```python
from build123d import *

# Parameters (mm, degrees)
BOSS_EXTRUDE1_DEPTH  = 3
SKETCH3_R            = 2.5
CUT_EXTRUDE1_DEPTH   = 4
LPATTERN1_COUNT      = 2
LPATTERN1_PITCH      = 40
LPATTERN1_COUNT_DIR2 = 2
LPATTERN1_PITCH_DIR2 = 20
SKETCH4_R            = 2.5
CUT_EXTRUDE2_DEPTH   = 4
LPATTERN2_COUNT      = 2
LPATTERN2_PITCH      = 40
FILLET1_R            = 5


with BuildPart() as part:
    # Sketch1 → Boss-Extrude1 (new body)
    with BuildSketch(Plane.XY):
        Polygon((0, 0), (20, 0), (60, 60), (60, 100), (0, 100), align=None)
    extrude(amount=BOSS_EXTRUDE1_DEPTH)

    # Sketch3 → Cut-Extrude1 (cut, through all)
    with BuildSketch(Plane.XY.offset(3)):
        with Locations((50, 90)):
            Circle(SKETCH3_R)
    cut_extrude1 = extrude(amount=-CUT_EXTRUDE1_DEPTH, mode=Mode.SUBTRACT)

    # LPattern1: Cut-Extrude1 2 × 2
    with Locations(*[(-i * LPATTERN1_PITCH, -j * LPATTERN1_PITCH_DIR2, 0) for i in range(LPATTERN1_COUNT) for j in range(LPATTERN1_COUNT_DIR2) if (i, j) != (0, 0)]):
        add(cut_extrude1, mode=Mode.SUBTRACT)

    # Sketch4 → Cut-Extrude2 (cut, through all)
    with BuildSketch(Plane.XY.offset(3)):
        with Locations((10, 10)):
            Circle(SKETCH4_R)
    cut_extrude2 = extrude(amount=-CUT_EXTRUDE2_DEPTH, mode=Mode.SUBTRACT)

    # LPattern2: Cut-Extrude2 ×2
    with Locations(*[(0, i * LPATTERN2_PITCH, 0) for i in range(1, LPATTERN2_COUNT)]):
        add(cut_extrude2, mode=Mode.SUBTRACT)

    # Fillet1
    fillet1_edges = [part.edges().sort_by_distance(p)[0] for p in [
        (0, 100, 1.5),
        (60, 100, 1.5),
        (60, 60, 1.5),
        (20, 0, 1.5),
        (0, 0, 1.5),
    ]]
    fillet(fillet1_edges, radius=FILLET1_R)


solid = part.part
```
Geometry check sheet. Reference: the model listing, model coordinates, mm. Give positions to 0.01 mm unless a question says otherwise; leave off trailing zeros. Write each loop counter-clockwise with the first axis right and the second up, starting at its lowest first coordinate (ties: lowest second). Pieces come first, ordered by that corner, then holes.
1) Section check B-B, the plane z = 2.35. Record the boundary of the cut face in (x, y).
2) Section check C-C, the plane y = 11.5. Record the boundary of the cut face in (x, z), and give its area (3 significant figures).
3) Material ranges on L1, parallel to Y at x = 10, z = 1; L2, parallel to Y at x = 50, z = 1.6; L3, parallel to X at y = 72, z = 0.8, recorded low to high.
4) Section check A-A, the plane y = 90. Record the boundary of the cut face in (x, z).
5) Release check for a two-part mould opening along Y. For faces 1 (the flat face through (23, 62, 0)), 2 (the cylindrical face through (2, 1, 2)), 3 (the cylindrical face through (9.67, 92.48, 1.52)) record: pulls with the +Y half, pulls with the -Y half, needs draft (parallel to the pull), parting line crosses it, or undercut.
6) Gauge pin test, flat end, axial feed: pin 1 (3 mm diameter, centred on x = 50, y = 70, fed in from -Z). Record the tip position at first contact, or that the pin passes through.
7) Section check D-D, the plane x = 40.5. Record the boundary of the cut face in (y, z).
Computed:
1. outline: (0, 5) arc R5 ccw to (5, 0) - (17.32, 0) arc R5 ccw to (21.48, 2.23) - (59.16, 58.74) arc R5 ccw to (60, 61.51) - (60, 95) arc R5 ccw to (55, 100) - (5, 100) arc R5 ccw to (0, 95) - close; hole circle Ø5 at (10, 10); hole circle Ø5 at (10, 50); hole circle Ø5 at (10, 70); hole circle Ø5 at (10, 90); hole circle Ø5 at (50, 70); hole circle Ø5 at (50, 90)
2. outline: (0, 0) - (8, 0) - (8, 3) - (0, 3) - close; (12, 0) - (27.67, 0) - (27.67, 3) - (12, 3) - close
2. area: 71.0 mm2
3. L1: y = 0 to 7.5, 12.5 to 47.5, 52.5 to 67.5, 72.5 to 87.5, 92.5 to 100
3. L2: y = 45 to 67.5, 72.5 to 87.5, 92.5 to 100
3. L3: x = 0 to 8.5, 11.5 to 48.5, 51.5 to 60
4. outline: (0, 0) - (7.5, 0) - (7.5, 3) - (0, 3) - close; (12.5, 0) - (47.5, 0) - (47.5, 3) - (12.5, 3) - close; (52.5, 0) - (60, 0) - (60, 3) - (52.5, 3) - close
5. face 1: needs draft
5. face 2: pulls with the -Y half
5. face 3: undercut
6. pin 1: passes through
7. outline: (30.75, 0) - (100, 0) - (100, 3) - (30.75, 3) - close
